from build123d import *

# Parameters (mm, degrees)
F0_R     = 11.5
F0_R_2   = 3.25
F1_DEPTH = 6
F0_R_3   = 1.5
F2_DEPTH = 3
F3_R     = 1


with BuildPart() as f1:
    # F0 (on Right) → F1 (new body)
    with BuildSketch(Plane.YZ):
        Circle(F0_R)
        with Locations((-5.3066, -5.3)):
            Circle(F0_R_2, mode=Mode.SUBTRACT)
        with Locations((5.3, -5.3066)):
            Circle(F0_R_2, mode=Mode.SUBTRACT)
        with Locations((-5.3, 5.3066)):
            Circle(F0_R_2, mode=Mode.SUBTRACT)
        with BuildLine():
            ThreePointArc((1.019757, 1.100043), (1.374706, 0.600152), (1.5, 0))
            ThreePointArc((1.5, 0), (-0.600093, -1.374732), (-1.019851, 1.099957))
            ThreePointArc((-1.019851, 1.099957), (-6.4e-05, 1.5), (1.019757, 1.100043))
        make_face(mode=Mode.SUBTRACT)
        with Locations((5.3066, 5.3)):
            Circle(F0_R_2, mode=Mode.SUBTRACT)
        with BuildLine():
            Line((-1.019851, 1.099957), (1.019757, 1.100043))
            ThreePointArc((1.019757, 1.100043), (-6.4e-05, 1.5), (-1.019851, 1.099957))
        make_face()
    extrude(amount=F1_DEPTH)

    # F0 (on Right) → F2 (join)
    with BuildSketch(Plane.YZ):
        with Locations((5.3066, 5.3)):
            Circle(F0_R_2)
        with Locations((5.3066, 5.3)):
            Circle(F0_R_3, mode=Mode.SUBTRACT)
        with Locations((-5.3066, -5.3)):
            Circle(F0_R_2)
        with Locations((-5.3066, -5.3)):
            Circle(F0_R_3, mode=Mode.SUBTRACT)
        with Locations((5.3, -5.3066)):
            Circle(F0_R_2)
        with Locations((5.3, -5.3066)):
            Circle(F0_R_3, mode=Mode.SUBTRACT)
        with Locations((-5.3, 5.3066)):
            Circle(F0_R_2)
        with Locations((-5.3, 5.3066)):
            Circle(F0_R_3, mode=Mode.SUBTRACT)
    extrude(amount=F2_DEPTH)

    # F3
    f3_edges = [f1.edges().sort_by_distance(p)[0] for p in [
        (0, -11.5, 0),
    ]]
    fillet(f3_edges, radius=F3_R)


solid = f1.part
Source: CAD feature listing. Evaluate the final solid. Frame: model axes, mm. A direction names the side the tool comes from. Coordinates: 2 decimals unless noted, no trailing zeros. Loops run counter-clockwise (first coordinate to the right, second up) from the corner with the lowest first, then second, coordinate; pieces in that order, holes last. Notation, with made-up numbers: (20.5, 81.5) - (29.5, 81.5) arc R15 cw to (29.5, 106.5) - close; hole circle Ø11 at (40.25, 48.5). An arc over 180 degrees is marked (long way). One line per question, with ' | ' between items.
1) First-contact query: P1, Ø2, axis at x = 4, y = -2, coming from the -Z side; P2, Ø4, axis at y = 5.3, z = -5.31, coming from the +X side; P3, Ø1.5, axis at x = 1, y = -8.5, coming from the -Z side. Flat tips, straight axial feed; report the tip coordinate or a pass-through.
Report:
P1: stops at z = -11.46 | P2: stops at x = 3 | P3: stops at z = -8.5
2) Line query: line 1 along Z through (x, y) = (0.6, 5.3); line 2 along Y through (x, z) = (4.7, 5); line 3 along Y through (x, z) = (0.9, -5). Output: solid intervals per line, ascending.
Report:
line 1: z = -10.11 to -6.81, -3.81 to 3.8, 6.8 to 10.11 | line 2: y = -10.36 to -8.54, -2.06 to 2.07, 8.54 to 10.36 | line 3: y = -10.35 to -6.78, -3.84 to 3.83, 6.77 to 10.35
3) Section B-B, the plane y = -5. Give the number of separate pieces and of enclosed holes in the cut face, then the cut area to 3 significant figures.
Report:
separate pieces: 3 | enclosed holes: 0 | area: 67.3 mm²
4) Section A-A, the plane x = 2.7. Return loops of the section in (y, z).
Report:
outline: circle Ø23 at (0, 0); hole circle Ø3 at (-5.31, -5.3); hole circle Ø3 at (-5.3, 5.31); hole (-1.02, 1.1) arc R1.5 ccw (long way) to (1.5, 0) arc R1.5 ccw to (1.02, 1.1) - close; hole circle Ø3 at (5.3, -5.31); hole circle Ø3 at (5.31, 5.3)
5) Set-up query: faces 1 (the face through (1.48, 3.8, -5.24)), 2 (the face through (3, 7, 5)). Return all of +Z, -Z, +X, -X, +Y, -Y with unobstructed straight access to the full face (end or side cutting, diameter ignored); none if empty.
Report:
face 1: +X, -X | face 2: +X
6) Pull-direction query (Z, two-part tool) for faces 3 (the face through (4.5, 8.4, 6.3)), 4 (the face through (1.48, 4.2, 6.31)), 5 (the face through (3.5, -1.5, 11.4)), 6 (the face through (0, 2, 0)); classes: released by +Z, released by -Z, zero draft, split by the parting line, or undercut.
Report:
face 3: undercut | face 4: undercut | face 5: split by the parting line | face 6: zero draft
